Check sheet for the modelled part. Datum: model origin and axes. Units: mm. Give positions to 0.01 mm unless a question says otherwise; leave off trailing zeros. Order: outer loops, then holes, each group sorted by start corner. A loop starts at its lowest first (then second) coordinate and runs counter-clockwise, first axis right, second up.
Item 1: Sectioned sample at C-C on z = -6. Record the boundary of the cut face in (x, y).
Item 2: Sectioned sample at A-A on y = 46. Record the boundary of the cut face in (x, z) (3 decimals).
Item 3: Sectioned sample at B-B on x = 37. Record the boundary of the cut face in (y, z).
Item 4: Material ranges on line 1 along X through (y, z) = (25, -33); line 2 along Z through (x, y) = (25, 58); line 3 along Y through (x, z) = (24, -43.5), recorded low to high.
Item 5: Gauge pin test, flat end, axial feed: P1, Ø12, axis at x = 40, z = -28, coming from the -Y side. Record the tip position at first contact, or that the pin passes through.
Item 6: Sectioned sample at D-D on z = -21. Record the boundary of the cut face in (x, y), and give its area (3 significant figures).
from build123d import *

# Parameters (mm, degrees)
SKETCH1_W               = 50.8
SKETCH1_H               = 50.8
BOSS_EXTRUDE1_DEPTH     = 76.2
CUT_EXTRUDE1_DEPTH      = 76.2
CUT_EXTRUDE2_REACH      = 106.727
CUT_EXTRUDE2_END_RADIUS = 17


with BuildPart() as part:
    # Sketch1 → Boss-Extrude1 (new body)
    with BuildSketch(Plane(origin=(0, 0, 0), x_dir=(1, 0, 0), z_dir=(0, 1, 0))):
        with Locations((25.4, 25.4)):
            Rectangle(SKETCH1_W, SKETCH1_H)
    extrude(amount=BOSS_EXTRUDE1_DEPTH)

    # Sketch2 → Cut-Extrude1 (cut)
    with BuildSketch(Plane(origin=(0, 0, -50.8), x_dir=(-1, 0, 0), z_dir=(0, 0, -1))):
        with BuildLine():
            ThreePointArc((-8.4, 25.4), (-37.42081528, 37.42081528), (-25.4, 8.4))
            Line((-25.4, 8.4), (-25.4, 25.4))
            Line((-25.4, 25.4), (-8.4, 25.4))
        make_face()
        with BuildLine():
            Line((-25.4, 25.4), (-25.4, 8.4))
            ThreePointArc((-25.4, 8.4), (-13.37918472, 13.37918472), (-8.4, 25.4))
            Line((-8.4, 25.4), (-25.4, 25.4))
        make_face()
    extrude(amount=-CUT_EXTRUDE1_DEPTH, mode=Mode.SUBTRACT)

    # Cut-Extrude2: up to this cylinder (the profile starts outside it)
    cut_extrude2_end = Plane(origin=(25.4, 25.4, -26.731477), z_dir=(0, 0, -1)) * Cylinder(CUT_EXTRUDE2_END_RADIUS, 257.437412, mode=Mode.PRIVATE)
    # Sketch3 → Cut-Extrude2 (cut, up to the surface)
    with BuildSketch(Plane(origin=(0, 76.2, 0), x_dir=(1, 0, 0), z_dir=(0, 1, 0)), mode=Mode.PRIVATE) as cut_extrude2_sk1:
        with BuildLine():
            ThreePointArc((41.275, 24.485623633), (36.625320151, 35.710943784), (25.4, 40.360623633))
            Line((25.4, 40.360623633), (25.4, 24.485623633))
            Line((25.4, 24.485623633), (9.525, 24.485623633))
            ThreePointArc((9.525, 24.485623633), (25.4, 8.610623633), (41.275, 24.485623633))
        make_face()
    cut_extrude2_tool1 = extrude(cut_extrude2_sk1.sketch, amount=-CUT_EXTRUDE2_REACH, mode=Mode.PRIVATE) - cut_extrude2_end
    add(cut_extrude2_tool1.solids().sort_by_distance((27.645853, 76.2, -22.239771))[0], mode=Mode.SUBTRACT)
    # Sketch3 → Cut-Extrude2 (cut, up to the surface)
    with BuildSketch(Plane(origin=(0, 76.2, 0), x_dir=(1, 0, 0), z_dir=(0, 1, 0)), mode=Mode.PRIVATE) as cut_extrude2_sk2:
        with BuildLine():
            Line((25.4, 24.485623633), (25.4, 40.360623633))
            ThreePointArc((25.4, 40.360623633), (14.174679849, 35.710943784), (9.525, 24.485623633))
            Line((9.525, 24.485623633), (25.4, 24.485623633))
        make_face()
    cut_extrude2_tool2 = extrude(cut_extrude2_sk2.sketch, amount=-CUT_EXTRUDE2_REACH, mode=Mode.PRIVATE) - cut_extrude2_end
    add(cut_extrude2_tool2.solids().sort_by_distance((18.662441, 76.2, -31.223183))[0], mode=Mode.SUBTRACT)
    # Sketch3 → Cut-Extrude2 (cut, up to the surface)
    with BuildSketch(Plane(origin=(0, 76.2, 0), x_dir=(1, 0, 0), z_dir=(0, 1, 0)), mode=Mode.PRIVATE) as cut_extrude2_sk3:
        with BuildLine():
            ThreePointArc((41.275, 24.485623633), (36.625320151, 35.710943784), (25.4, 40.360623633))
            Line((25.4, 40.360623633), (25.4, 24.485623633))
            Line((25.4, 24.485623633), (9.525, 24.485623633))
            ThreePointArc((9.525, 24.485623633), (25.4, 8.610623633), (41.275, 24.485623633))
        make_face()
    cut_extrude2_tool3 = extrude(cut_extrude2_sk3.sketch, amount=-CUT_EXTRUDE2_REACH, mode=Mode.PRIVATE) - cut_extrude2_end
    add(cut_extrude2_tool3.solids().sort_by_distance((27.645853, 76.2, -22.239771))[0], mode=Mode.SUBTRACT)
    # Sketch3 → Cut-Extrude2 (cut, up to the surface)
    with BuildSketch(Plane(origin=(0, 76.2, 0), x_dir=(1, 0, 0), z_dir=(0, 1, 0)), mode=Mode.PRIVATE) as cut_extrude2_sk4:
        with BuildLine():
            Line((25.4, 24.485623633), (25.4, 40.360623633))
            ThreePointArc((25.4, 40.360623633), (14.174679849, 35.710943784), (9.525, 24.485623633))
            Line((9.525, 24.485623633), (25.4, 24.485623633))
        make_face()
    cut_extrude2_tool4 = extrude(cut_extrude2_sk4.sketch, amount=-CUT_EXTRUDE2_REACH, mode=Mode.PRIVATE) - cut_extrude2_end
    add(cut_extrude2_tool4.solids().sort_by_distance((18.662441, 76.2, -31.223183))[0], mode=Mode.SUBTRACT)


solid = part.part
Report:
1. outline: (0, 0) - (50.8, 0) - (50.8, 76.2) - (0, 76.2) - close; hole circle Ø34 at (25.4, 25.4)
2. outline: (0, -50.8) - (50.8, -50.8) - (50.8, 0) - (0, 0) - close; hole circle Ø31.75 at (25.4, -24.486)
3. outline: (0, -50.8) - (12.97, -50.8) - (12.97, 0) - (0, 0) - close; (37.83, -50.8) - (76.2, -50.8) - (76.2, -35.32) - (37.83, -35.32) - close; (37.83, -13.65) - (76.2, -13.65) - (76.2, 0) - (37.83, 0) - close
4. line 1: x = 0 to 8.4, 42.4 to 50.8
4. line 2: z = -50.8 to -40.36, -8.62 to 0
4. line 3: y = 0 to 8.46, 42.34 to 76.2
5. P1: stops at y = 0
6. outline: (0, 0) - (50.8, 0) - (50.8, 76.2) - (40.89, 76.2) - (40.89, 32.41) arc R17 cw (long way) to (9.91, 32.41) - (9.91, 76.2) - (0, 76.2) - close
6. area: 1,830 mm2
